Verification items for the finished model (mm, model axes). Coordinates: 2 decimals unless noted, no trailing zeros. Order: outer loops, then holes, each group sorted by start corner. A loop starts at its lowest first (then second) coordinate and runs counter-clockwise, first axis right, second up. Notation, with made-up numbers: M 79.5,-8 L 106.5,-8 A21 ccw 106.5,4 Z; hole C 62.5,-8 d3. An arc over 180 degrees is marked long. Answer as a JSON object with one key per item and string values. Group by question number.
(1) Cross-section at C-C (x = 115). Enter the section's corners in (y, z), plus the area to 3 significant figures.
(2) Cross-section at B-B (z = 0.75). Count the separate pieces of the cut face and the enclosed holes in it, plus the area to 3 significant figures.
(3) Material ranges on line 1 (Y direction, x = -120.65, z = 0); line 2 (X direction, y = 30, z = 4.25); line 3 (X direction, y = -1, z = 4.25), recorded low to high.
(4) Gauge pin test, flat ends, axial feed: pin 1 Ø3 at (y, z) = (-20, 3) entering from +X; pin 2 Ø10 at (x, y) = (-174.625, 0) entering from +Z; pin 3 Ø6 at (x, z) = (109, 1.5) entering from -Y; pin 4 Ø3 at (x, z) = (90.5, 0) entering from +Y. Record the tip position at first contact, or that the pin passes through.
(5) Cross-section at A-A (x = 56.5). Enter the section's corners in (y, z).
from build123d import *

# Parameters (mm, degrees)
F0_R     = 6.35
F0_R_2   = 7.9375
F1_DEPTH = 6.35
F2_R     = 11.1125
F3_DEPTH = 3.175


with BuildPart() as f1:
    # F0 (on Top) → F1 (new body, symmetric)
    with BuildSketch(Plane.XY):
        with BuildLine():
            ThreePointArc((-120.65, -38.1), (-105.0957401333, -34.7803824016), (-92.2519366858, -25.4))
            ThreePointArc((-92.2519366858, -25.4), (-82.55, 0), (-92.2519366858, 25.4))
            ThreePointArc((-92.2519366858, 25.4), (-105.0957401333, 34.7803824016), (-120.65, 38.1))
            Line((-120.65, 38.1), (-174.625, 38.1))
            ThreePointArc((-174.625, 38.1), (-190.1792598667, 34.7803824016), (-203.0230633142, 25.4))
            ThreePointArc((-203.0230633142, 25.4), (-210.2169668893, 13.5949215867), (-212.725, -7.2e-08))
            ThreePointArc((-212.725, -7.2e-08), (-210.2169668636, -13.594921654), (-203.0230633142, -25.4))
            ThreePointArc((-203.0230633142, -25.4), (-190.1792598667, -34.7803824016), (-174.625, -38.1))
            Line((-174.625, -38.1), (-120.65, -38.1))
        make_face()
        with Locations((-174.625, 0)):
            Circle(F0_R, mode=Mode.SUBTRACT)
        with Locations((-120.65, 0)):
            Circle(F0_R, mode=Mode.SUBTRACT)
        with BuildLine():
            Line((-92.2519366858, -25.4), (158.9269366858, -25.4))
            ThreePointArc((158.9269366858, -25.4), (149.225, 0), (158.9269366858, 25.4))
            Line((158.9269366858, 25.4), (80.0710946124, 25.4))
            ThreePointArc((80.0710946124, 25.4), (84.2698408134, 17.8971594032), (85.725, 9.4234))
            ThreePointArc((85.725, 9.4234), (51.8512405968, -14.5214408134), (40.5789053876, 25.4))
            Line((40.5789053876, 25.4), (-92.2519366858, 25.4))
            ThreePointArc((-92.2519366858, 25.4), (-82.55, 0), (-92.2519366858, -25.4))
        make_face()
        with BuildLine():
            ThreePointArc((158.9269366858, 25.4), (149.225, 0), (158.9269366858, -25.4))
            ThreePointArc((158.9269366858, -25.4), (200.9199216204, -35.5919668765), (225.425, 0))
            ThreePointArc((225.425, 0), (200.9199216204, 35.5919668765), (158.9269366858, 25.4))
        make_face()
        with Locations((187.325, 0)):
            Circle(F0_R, mode=Mode.SUBTRACT)
        with BuildLine():
            ThreePointArc((85.725, 9.4234), (84.2698408134, 17.8971594032), (80.0710946124, 25.4))
            Line((80.0710946124, 25.4), (40.5789053876, 25.4))
            ThreePointArc((40.5789053876, 25.4), (51.8512405968, -14.5214408134), (85.725, 9.4234))
        make_face()
        with Locations((60.325, 9.4234)):
            Circle(F0_R_2, mode=Mode.SUBTRACT)
        with BuildLine():
            Line((40.5789053876, 25.4), (80.0710946124, 25.4))
            ThreePointArc((80.0710946124, 25.4), (60.325, 34.8234), (40.5789053876, 25.4))
        make_face()
    extrude(amount=F1_DEPTH, both=True)

    # F2 (on face) → F3 (cut)
    with BuildSketch(Plane.XY.offset(6.35)):
        with Locations((-174.625, 0)):
            Circle(F2_R)
    extrude(amount=-F3_DEPTH, mode=Mode.SUBTRACT)


solid = f1.part
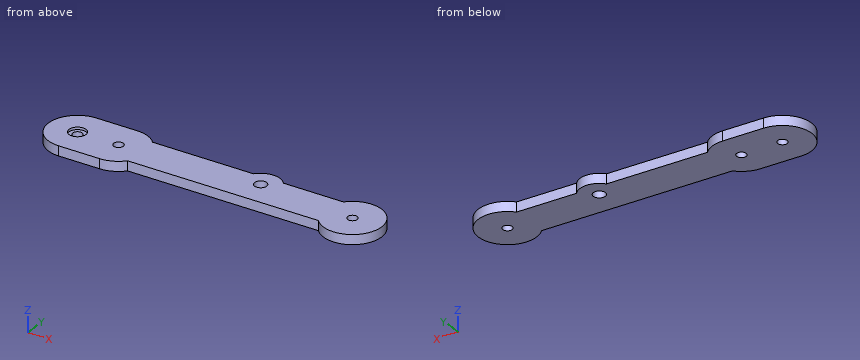
Taken from the geometry:
{
 "1": {"outline": "M -25.4,-6.35 L 25.4,-6.35 L 25.4,6.35 L -25.4,6.35 Z", "area": "645 mm²"},
 "2": {"separate pieces": "1", "enclosed holes": "4", "area": "25,000 mm²"},
 "3": {"line 1": "y = -38.1 to -6.35, 6.35 to 38.1", "line 2": "x = -198.11 to -97.16, 45.43 to 75.22, 163.84 to 210.81", "line 3": "x = -212.71 to -185.69, -163.56 to -126.92, -114.38 to 181.05, 193.6 to 225.41"},
 "4": {"pin 1": "stops at x = 220.63", "pin 2": "passes through", "pin 3": "stops at y = -25.4", "pin 4": "stops at y = 25.4"},
 "5": {"outline": "M -25.4,-6.35 L 2.47,-6.35 L 2.47,6.35 L -25.4,6.35 Z; M 16.38,-6.35 L 34.53,-6.35 L 34.53,6.35 L 16.38,6.35 Z"}
}
